```python
from build123d import *

# Parameters (mm, degrees)
F1_DEPTH = 10
F2_DEPTH = 4.7


with BuildPart() as f1:
    # F0 (on Top) → F1 (new body)
    with BuildSketch(Plane.XY):
        with BuildLine():
            ThreePointArc((0, -3.1), (2.1920310217, -2.1920310217), (3.1, 0))
            ThreePointArc((3.1, 0), (2.9328670446, 1.0041368924), (2.4494897428, 1.9))
            Line((2.4494897428, 1.9), (0, 1.9))
            Line((0, 1.9), (0, 1.1))
            ThreePointArc((0, 1.1), (0.4974937186, 0.9810708435), (0.8874119675, 0.65))
            ThreePointArc((0.8874119675, 0.65), (1.0455030283, 0.3419406643), (1.1, 0))
            ThreePointArc((1.1, 0), (0.7778174593, -0.7778174593), (0, -1.1))
            Line((0, -1.1), (0, -3.1))
        make_face()
        with BuildLine():
            ThreePointArc((-2.4494897428, 1.9), (-2.7838821814, -1.3638181697), (0, -3.1))
            Line((0, -3.1), (0, -1.1))
            ThreePointArc((0, -1.1), (-0.9810708435, -0.4974937186), (-0.8874119675, 0.65))
            ThreePointArc((-0.8874119675, 0.65), (-0.4974937186, 0.9810708435), (0, 1.1))
            Line((0, 1.1), (0, 1.9))
            Line((0, 1.9), (-2.4494897428, 1.9))
        make_face()
        with BuildLine():
            ThreePointArc((0.8874119675, 0.65), (0.4974937186, 0.9810708435), (0, 1.1))
            Line((0, 1.1), (0, 0.65))
            Line((0, 0.65), (0.8874119675, 0.65))
        make_face()
        with BuildLine():
            Line((0, 0.65), (0, 1.1))
            ThreePointArc((0, 1.1), (-0.4974937186, 0.9810708435), (-0.8874119675, 0.65))
            Line((-0.8874119675, 0.65), (0, 0.65))
        make_face()
    extrude(amount=F1_DEPTH)

    # F0 (on Top) → F2 (join)
    with BuildSketch(Plane.XY):
        with BuildLine():
            Line((0, 1.9), (2.4494897428, 1.9))
            ThreePointArc((2.4494897428, 1.9), (0, 3.1), (-2.4494897428, 1.9))
            Line((-2.4494897428, 1.9), (0, 1.9))
        make_face()
    extrude(amount=F2_DEPTH)


solid = f1.part
```
Geometry: final body of the model. Coordinates: model frame, mm. A direction names the side the tool comes from. Coordinates: 2 decimals unless noted, no trailing zeros. Write each loop counter-clockwise with the first axis right and the second up, starting at its lowest first coordinate (ties: lowest second). Pieces come first, ordered by that corner, then holes. Notation, with made-up numbers: M -16,-28 L 8,-28 A29 ccw 8,-5 Z; hole C 72.5,85 d7. An arc over 180 degrees is marked long. Use CSV: the item, a comma, the result in double quotes. Start each with the question number.
1. Cut plane A-A on z = 1. Return the cut outline in (x, y), plus the area to 3 significant figures.
2. Cut plane C-C on z = 6.75. Return the cut outline in (x, y).
3. Reachability of faces 4 (the face through (0, 2.4, 4.7)), 5 (the face through (1, -1, 10)) from +Z, -Z, +X, -X, +Y, -Y: full face, straight path, thin tool, end or side. Return the list, or none.
4. Cut plane B-B on y = -0.25. Return the cut outline in (x, z), plus the area to 3 significant figures.
5. Mould query, pull axis Y, two halves, no side actions, for faces 1 (the face through (0, 0.65, 5)), 2 (the face through (0, 1, 0)), 3 (the face through (0, 1.9, 7)). Classes: pulls with the +Y half, pulls with the -Y half, needs draft (parallel to the pull), parting line crosses it, or undercut.
6. First-contact query: P1, Ø1, axis at x = -1, y = 2.5, coming from the +Z side. Flat tip, straight axial feed; report the tip coordinate or a pass-through.
7. Cut plane D-D on x = 2. Return the cut outline in (y, z), plus the area to 3 significant figures.
8. Ray query, probe 1 along X at (y, z) = (-0.5, 4); probe 2 along X at (y, z) = (-1, 9.25); probe 3 along Y at (x, z) = (0.25, 1). Return the intervals inside material, ascending.
Entries:
1,outline,"C 0,0 d6.2; hole M -0.89,0.65 A1.1 ccw long 0.89,0.65 Z"
1,area,"26.9 mm²"
2,outline,"M -2.45,1.9 A3.1 ccw long 2.45,1.9 Z; hole M -0.89,0.65 A1.1 ccw long 0.89,0.65 Z"
3,face 4,"+Z, +X, -X, +Y"
3,face 5,"+Z, +X, -X, +Y, -Y"
4,outline,"M -3.09,0 L -1.07,0 L -1.07,10 L -3.09,10 Z; M 1.07,0 L 3.09,0 L 3.09,10 L 1.07,10 Z"
4,area,"40.4 mm²"
5,face 1,"undercut"
5,face 2,"needs draft"
5,face 3,"pulls with the +Y half"
6,P1,"z = 4.7"
7,outline,"M -2.37,0 L 2.37,0 L 2.37,4.7 L 1.9,4.7 L 1.9,10 L -2.37,10 Z"
7,area,"44.9 mm²"
8,probe 1,"-3.06 to -0.98, 0.98 to 3.06"
8,probe 2,"-2.93 to -0.46, 0.46 to 2.93"
8,probe 3,"-3.09 to -1.07, 0.65 to 3.09"
